Autodesk Inventor part; units mm, degrees
ref_plane "YZ Plane" through (0, 0, 0) normal (1, 0, 0) x (0, 1, 0)
ref_plane "XZ Plane" through (0, 0, 0) normal (0, 1, 0) x (-1, 0, 0)
ref_plane "XY Plane" through (0, 0, 0) normal (0, 0, 1) x (1, 0, 0)
sketch "スケッチ1" plane through (0, 0, 0) normal (0, 0, 1) x (1, 0, 0)
  line L0 (75, -52.5) -> (-75, -52.5)
  line L1 (-75, -52.5) -> (-75, 52.5)
  line L2 (-75, 52.5) -> (75, 52.5)
  line L3 (75, 52.5) -> (75, -52.5)
  line L4 (75, -52.5) -> (-75, 52.5) construction
  line L5 (-75, -52.5) -> (75, 52.5) construction
  line L6 (76.5, -54) -> (-76.5, -54)
  line L7 (-76.5, -54) -> (-76.5, 54)
  line L8 (-76.5, 54) -> (76.5, 54)
  line L9 (76.5, 54) -> (76.5, -54)
  line L10 (76.5, -54) -> (-76.5, 54) construction
  line L11 (-76.5, -54) -> (76.5, 54) construction
  point P0 (0, 0)
  dimension "d0" = 150
  dimension "d1" = 105
  dimension "d4" = 153
  dimension "d5" = 108
extrude "押し出し1" add sketch "スケッチ1" along normal blind 40
extrude "押し出し2" add sketch "スケッチ1" along normal blind 3 contours L0 L1 L2 L3
fillet "フィレット3" radius 3 4 edges at (-76.5, 54, 20) (-76.5, -54, 20) (76.5, -54, 20) (76.5, 54, 20)
fillet "フィレット3" radius 3 4 edges at (-75, 52.5, 21.5) (75, 52.5, 21.5) (-75, -52.5, 21.5) (75, -52.5, 21.5)
properties part number "water_bowl"
Verification items for the finished model (mm, model axes). A direction names the side the tool comes from. Coordinates: 2 decimals unless noted, no trailing zeros. Loops run counter-clockwise (first coordinate to the right, second up) from the corner with the lowest first, then second, coordinate; pieces in that order, holes last. Notation, with made-up numbers: (-5.75, -32) - (43.25, -32) arc R24 ccw to (43.25, -22) - close; hole circle Ø11 at (29.5, -36). An arc over 180 degrees is marked (long way). Answer as a JSON object with one key per item and string values.
(1) Mould release check, pull along Y, two halves, no side actions. Record for faces 1 (the cylindrical face through (75.6, -53.14, 20.28)), 2 (the flat face through (75, 1, 21)), 3 (the cylindrical face through (75.64, 53.1, 20.28)): pulls with the +Y half, pulls with the -Y half, needs draft (parallel to the pull), parting line crosses it, or undercut.
Response:
{"face 1": "pulls with the -Y half", "face 2": "undercut", "face 3": "pulls with the +Y half"}
(2) Cross-section at C-C, the plane x = 9.5. Record the boundary of the cut face in (y, z).
Response:
{"outline": "(-54, 0) - (54, 0) - (54, 40) - (52.5, 40) - (52.5, 3) - (-52.5, 3) - (-52.5, 40) - (-54, 40) - close"}
(3) Access from +Z, -Z, +X, -X, +Y, -Y to the whole of each face (thin tool, end or side, straight path). Record for faces 4 (the cylindrical face through (74.14, 51.6, 21.76)), 5 (the flat face through (-1, 54, 20)).
Response:
{"face 4": "+Z", "face 5": "+Z, -Z, +X, -X, +Y"}
(4) Cross-section at B-B, the plane z = 10.5. Record the boundary of the cut face in (x, y).
Response:
{"outline": "(-76.5, -51) arc R3 ccw to (-73.5, -54) - (73.5, -54) arc R3 ccw to (76.5, -51) - (76.5, 51) arc R3 ccw to (73.5, 54) - (-73.5, 54) arc R3 ccw to (-76.5, 51) - close; hole (-75, -49.5) arc R3 ccw to (-72, -52.5) - (72, -52.5) arc R3 ccw to (75, -49.5) - (75, 49.5) arc R3 ccw to (72, 52.5) - (-72, 52.5) arc R3 ccw to (-75, 49.5) - close"}
(5) Go/stop test with a flat-tipped pin: pin 1 Ø5 at (x, y) = (7.5, -22.5) entering from -Z. Record where the tip stops, or that it passes through.
Response:
{"pin 1": "stops at z = 0"}
(6) Cross-section at A-A, the plane y = -44.5. Record the boundary of the cut face in (x, z).
Response:
{"outline": "(-76.5, 0) - (76.5, 0) - (76.5, 40) - (75, 40) - (75, 3) - (-75, 3) - (-75, 40) - (-76.5, 40) - close"}
(7) Scan lines: line 1 along X through (y, z) = (0, 22.5); line 2 along Y through (x, z) = (59, 13.5); line 3 along Z through (x, y) = (19.5, 37). Record each from-to range of solid material in increasing order.
Response:
{"line 1": "x = -76.5 to -75, 75 to 76.5", "line 2": "y = -54 to -52.5, 52.5 to 54", "line 3": "z = 0 to 3"}
